Here's how the part is built. I have some questions about the finished solid (model axes, mm). Face numbers are marked on the shaded views. A direction names the side the tool comes from. Coordinates: 2 decimals unless noted, no trailing zeros. Write each loop counter-clockwise with the first axis right and the second up, starting at its lowest first coordinate (ties: lowest second). Pieces come first, ordered by that corner, then holes. Notation, with made-up numbers: (60.5, 52.25) -> (98.5, 52.25) arc R23 ccw to (98.5, 71.25) -> close; hole circle Ø5 at (-30.75, -6). An arc over 180 degrees is marked (long way). Answer in a Markdown table with one row per item. Add a question column.
from build123d import *

# Parameters (mm, degrees)
ESQUISSE1_W             = 56
ESQUISSE1_H             = 40
BOSS_EXTRU_1_DEPTH      = 15.3
ESQUISSE2_R             = 20
BOSS_EXTRU_2_DEPTH      = 13
ESQUISSE5_R             = 1.4
ENL_V_MAT_EXTRU_1_DEPTH = 5
ESQUISSE6_R             = 16
ENL_V_MAT_EXTRU_2_DEPTH = 28.1
ESQUISSE3_R             = 2.55
ENL_V_MAT_EXTRU_3_DEPTH = 28


with BuildPart() as part:
    # Esquisse1 → Boss.-Extru.1 (new body)
    with BuildSketch(Plane.XY):
        Rectangle(ESQUISSE1_W, ESQUISSE1_H)
    extrude(amount=BOSS_EXTRU_1_DEPTH)

    # Esquisse2 → Boss.-Extru.2 (add)
    with BuildSketch(Plane.XY.offset(15.3)):
        with Locations(Location((0, 0, 0), (0, 0, 270))):
            Circle(ESQUISSE2_R)
    extrude(amount=BOSS_EXTRU_2_DEPTH)

    # Esquisse5 → Enlèv. mat.-Extru.1 (cut)
    with BuildSketch(Plane(origin=(0, 20, 0), x_dir=(1, 0, 0), z_dir=(0, 1, 0))):
        with Locations(Location((-21.45, -7.6, 0), (0, 0, 180))):
            Circle(ESQUISSE5_R)
        with Locations(Location((21.45, -7.6, 0), (0, 0, 180))):
            Circle(ESQUISSE5_R)
    extrude(amount=-ENL_V_MAT_EXTRU_1_DEPTH, mode=Mode.SUBTRACT)

    # Esquisse6 → Enlèv. mat.-Extru.2 (cut)
    with BuildSketch(Plane(origin=(0, 0, 0), x_dir=(-1, 0, 0), z_dir=(0, 0, -1))):
        Circle(ESQUISSE6_R)
    extrude(amount=-ENL_V_MAT_EXTRU_2_DEPTH, mode=Mode.SUBTRACT)

    # Esquisse3 → Enlèv. mat.-Extru.3 (cut)
    with BuildSketch(Plane.XY.offset(28.3)):
        Circle(ESQUISSE3_R)
    extrude(amount=-ENL_V_MAT_EXTRU_3_DEPTH, mode=Mode.SUBTRACT)


solid = part.part
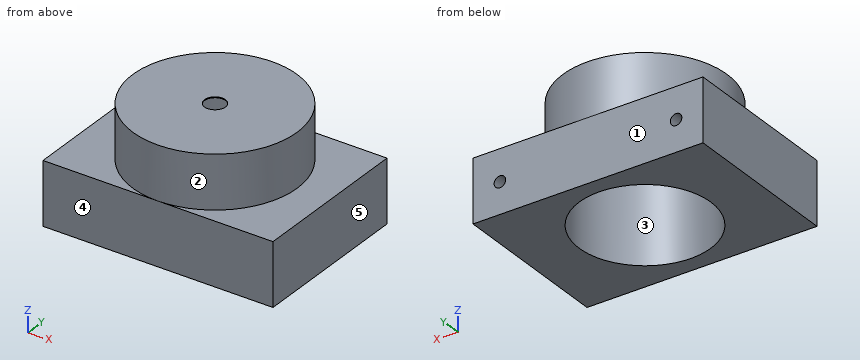
Q1. I'm going to push flat-ended pins straight in: P1, Ø8, axis at x = -3.5, y = -6, coming from the -Z side; P2, Ø1.4, axis at x = 21.5, z = 8, coming from the +Y side. Where does each tip first touch, or does it pass through?
Q2. Imagine slicing it at C-C on z = 7.6. Please give me the cut outline in (x, y).
Q3. Imagine slicing it at B-B on x = 21.45. Please give me the cut outline in (y, z).
Q4. If we mould it in two halves opening along X, with no side actions, what happens to the marked faces 3, 4 and 5? For each: pulls with the +X half, pulls with the -X half, needs draft (parallel to the pull), parting line crosses it, or undercut.
Q5. Imagine slicing it at A-A on y = 0. Please give me the cut outline in (x, z), plus the area to 3 significant figures.
Q6. For the marked faces 1 and 2, which set-ups out of +Z, -Z, +X, -X, +Y, -Y let a thin tool reach every point of the face, with its end or its side?
Q7. I need wall thicknesses on line 1 (Z direction, x = 21.45, y = 17.1); line 2 (X direction, y = -0.5, z = 18.5); line 3 (Y direction, x = 0, z = 28.25). Which ranges of each line are inside material? Lowest first, please. Write a range as [from, to].
Q8. Imagine slicing it at D-D on x = -1.5. Please give me the cut outline in (y, z), plus the area to 3 significant figures.
Result sheet:
| question | item | result |
|---|---|---|
| 1 | P1 | stops at z = 28.1 |
| 1 | P2 | stops at y = 15 |
| 2 | outline | (-28, -20) -> (28, -20) -> (28, 20) -> (22.85, 20) -> (22.85, 15) -> (20.05, 15) -> (20.05, 20) -> (-20.05, 20) -> (-20.05, 15) -> (-22.85, 15) -> (-22.85, 20) -> (-28, 20) -> close; hole circle Ø32 at (0, 0) |
| 3 | outline | (-20, 0) -> (20, 0) -> (20, 6.2) -> (15, 6.2) -> (15, 9) -> (20, 9) -> (20, 15.3) -> (-20, 15.3) -> close |
| 4 | face 3 | undercut |
| 4 | face 4 | needs draft |
| 4 | face 5 | pulls with the +X half |
| 5 | outline | (-28, 0) -> (-16, 0) -> (-16, 28.1) -> (-2.55, 28.1) -> (-2.55, 28.3) -> (-20, 28.3) -> (-20, 15.3) -> (-28, 15.3) -> close; (2.55, 28.1) -> (16, 28.1) -> (16, 0) -> (28, 0) -> (28, 15.3) -> (20, 15.3) -> (20, 28.3) -> (2.55, 28.3) -> close |
| 5 | area | 477 mm^2 |
| 6 | face 1 | +Z, -Z, +X, -X, +Y |
| 6 | face 2 | +Z |
| 7 | line 1 | z = [0, 6.2], [9, 15.3] |
| 7 | line 2 | x = [-19.99, -15.99], [15.99, 19.99] |
| 7 | line 3 | y = [-20, -2.55], [2.55, 20] |
| 8 | outline | (-20, 0) -> (-15.93, 0) -> (-15.93, 28.1) -> (-2.06, 28.1) -> (-2.06, 28.3) -> (-19.94, 28.3) -> (-19.94, 15.3) -> (-20, 15.3) -> close; (2.06, 28.1) -> (15.93, 28.1) -> (15.93, 0) -> (20, 0) -> (20, 15.3) -> (19.94, 15.3) -> (19.94, 28.3) -> (2.06, 28.3) -> close |
| 8 | area | 234 mm^2 |
